The listing builds one solid part. Answer for the finished solid, in the listing's coordinates (mm). Coordinates: 2 decimals unless noted, no trailing zeros. Order: outer loops, then holes, each group sorted by start corner. A loop starts at its lowest first (then second) coordinate and runs counter-clockwise, first axis right, second up. Notation, with made-up numbers: (59.25, 58) -> (80.25, 58) arc R16 cw to (80.25, 64) -> close; hole circle Ø7 at (15.5, 33). An arc over 180 degrees is marked (long way). One line per question, with ' | ' between items.
from build123d import *

# Parameters (mm, degrees)
CUT_EXTRUDE1_DEPTH = 0.8


with BuildPart() as part:
    # Sketch2 → Revolve1 (revolve)
    with BuildSketch(Plane.XY):
        Polygon((0, 0), (0, 2.5), (0.15, 2.5), (1.4, 1.25), (5.75, 1.25), (6, 1), (6, 0), align=None)
    revolve(axis=Axis((-2.281841559, 0, 0), (1, 0, 0)))

    # Sketch3 → Cut-Extrude1 (cut)
    with BuildSketch(Plane.ZY):
        Polygon((0.433012702, -0.75), (0.866025404, 0), (0.433012702, 0.75), (-0.433012702, 0.75), (-0.866025404, 0), (-0.433012702, -0.75), align=None)
    extrude(amount=-CUT_EXTRUDE1_DEPTH, mode=Mode.SUBTRACT)


solid = part.part
Item 1: Find the intervals of material crossed by L1, parallel to X at y = -0.3, z = 0.2; L2, parallel to Z at x = 3.1, y = 1; L3, parallel to X at y = 0.1, z = 1.8, in increasing order.
Computed values:
L1: x = 0.8 to 6 | L2: z = -0.75 to 0.75 | L3: x = 0 to 0.85
Item 2: Section C-C, the plane x = 3.15 is taken. Give the vertices of the cut face in (y, z), plus the area to 3 significant figures.
Computed values:
outline: circle Ø2.5 at (0, 0) | area: 4.91 mm^2
Item 3: Determine the mould class of faces 1 (the face through (3.61, -0.27, -1.22)), 2 (the face through (0.8, 0, 0)), 3 (the face through (6, 0, 0)) for opening direction Y: pulls with the +Y half, pulls with the -Y half, needs draft (parallel to the pull), parting line crosses it, or undercut.
Computed values:
face 1: parting line crosses it | face 2: undercut | face 3: needs draft
Item 4: Section A-A, the plane z = 0 is taken. Give the vertices of the cut face in (x, y), plus the area to 3 significant figures.
Computed values:
outline: (0, -2.5) -> (0.15, -2.5) -> (1.4, -1.25) -> (5.75, -1.25) -> (6, -1) -> (6, 1) -> (5.75, 1.25) -> (1.4, 1.25) -> (0.15, 2.5) -> (0, 2.5) -> (0, 0.75) -> (0.8, 0.75) -> (0.8, -0.75) -> (0, -0.75) -> close | area: 15.7 mm^2
Item 5: Each of these flat-tipped pins is pushed along its axis until it touches: pin 1 Ø2 at (x, y) = (1, 1.5) entering from -Z; pin 2 Ø2 at (x, y) = (4.5, -1) entering from +Z. Where does it stop, or does it pass through?
Computed values:
pin 1: stops at z = -2.3 | pin 2: stops at z = 1.25
Item 6: Section B-B, the plane x = 0.7 is taken. Give the vertices of the cut face in (y, z).
Computed values:
outline: circle Ø3.9 at (0, 0); hole (-0.75, -0.43) -> (0, -0.87) -> (0.75, -0.43) -> (0.75, 0.43) -> (0, 0.87) -> (-0.75, 0.43) -> close
